```python
from build123d import *

# Parameters (mm, degrees)
F0_R         = 18.561525572
F1_DEPTH     = 25
F2_T         = -2.5
F3_W         = 33.1976041198
F3_H         = 14.1467070207
F4_DEPTH     = 25
F5_T         = -2.5
F7_DEPTH     = 3
F9_DEPTH     = 3
F10_T1_DEPTH = 58.1976041198
F11_T1_DEPTH = 58.1976041198


# Not quite as in the source:
# - a fillet or chamfer that OpenCascade refuses, or shapes differently, is made with other operations: its cross-section is extruded or revolved along the edge and cut away or added
# - a shell that OpenCascade refuses in one call is made with other operations: the cavity is built on its own and cut out


with BuildPart() as f1:
    # F0 (on Top) → F1 (new body)
    with BuildSketch(Plane.XY):
        Circle(F0_R)
    extrude(amount=F1_DEPTH)

    # F2
    f2_openings = [f1.faces().sort_by_distance(p)[0] for p in [
        (0, 0, 25),
        (0, 0, 0),
    ]]
    offset(amount=F2_T, openings=f2_openings)

    # F3 (on Top) → F4 (join)
    with BuildSketch(Plane.XY):
        with Locations((0.0943113118, 0.2829344012)):
            Rectangle(F3_W, F3_H)
    extrude(amount=-F4_DEPTH)

    # F5: a shell. OpenCascade refuses it in one call, so the cavity is built on its own and cut out:
    # the body offset inwards by the wall thickness, plus a prism from it out through each open face.
    f5_core = offset(f1.part, amount=F5_T, mode=Mode.PRIVATE)
    f5_exits = [f5_core.faces().sort_by_distance(p)[0] for p in [
        (0.094311, 0.282934, -22.5),
        (0.094311, 0.282934, -2.5),
    ]]
    add(f5_core, mode=Mode.SUBTRACT)
    extrude(f5_exits, amount=-F5_T, mode=Mode.SUBTRACT)

    # F6 (on Top) → F7 (join)
    with BuildSketch(Plane.XY):
        with BuildLine():
            Line((16.6573040187, -6.7166290246), (-16.5601819754, -6.760219112))
            ThreePointArc((-16.5601819754, -6.760219112), (0.0631717454, -17.8724120589), (16.6573040187, -6.7166290246))
        make_face()
    extrude(amount=F7_DEPTH)

    # F8 (on Top) → F9 (join)
    with BuildSketch(Plane.XY):
        with BuildLine():
            Line((-16.4011158049, 7.3119108565), (16.5623016655, 7.2848270647))
            ThreePointArc((16.5623016655, 7.2848270647), (0.0891507264, 17.7139786602), (-16.4011158049, 7.3119108565))
        make_face()
    extrude(amount=F9_DEPTH)

    # F10: fillet of radius 5 on 1 edges, made by hand

    # F10_s2 → F10_t1 (cut)
    with BuildSketch(Plane.YZ.offset(-29.004490748)):
        with BuildLine():
            ThreePointArc((-1.7904191092, -25), (-5.3259530151, -23.5355339059), (-6.7904191092, -20))
            Line((-6.7904191092, -20), (-6.7904191092, -25))
            Line((-6.7904191092, -25), (-1.7904191092, -25))
        make_face()
    extrude(amount=F10_T1_DEPTH, mode=Mode.SUBTRACT)

    # F11: fillet of radius 5 on 1 edges, made by hand

    # F11_s2 → F11_t1 (cut)
    with BuildSketch(Plane.YZ.offset(-29.004490748)):
        with BuildLine():
            ThreePointArc((7.3562879115, -20), (5.8918218175, -23.5355339059), (2.3562879115, -25))
            Line((2.3562879115, -25), (7.3562879115, -25))
            Line((7.3562879115, -25), (7.3562879115, -20))
        make_face()
    extrude(amount=F11_T1_DEPTH, mode=Mode.SUBTRACT)


solid = f1.part
```
Here's how the part is built. I have some questions about the finished solid (model axes, mm). A direction names the side the tool comes from. Round coordinates to 2 decimals unless told otherwise and drop trailing zeros. Order: outer loops, then holes, each group sorted by start corner. A loop starts at its lowest first (then second) coordinate and runs counter-clockwise, first axis right, second up. Notation, with made-up numbers: (76, 50) -> (103, 50) arc R17 ccw to (103, 58) -> close; hole circle Ø5 at (59.25, 54). An arc over 180 degrees is marked (long way). Use a Markdown table: item, result. Add a question column.
(1) Suppose I cut it at B-B, the plane z = -16. Please give me the cut outline in (x, y).
(2) If we mould it in two halves opening along Y, with no side actions, what happens to faces 1 (the face through (-0.138, -5.854, -22.913)), 2 (the face through (-0.1, 6.5, -22.8)), 3 (the face through (-11, 12, 25)), 4 (the face through (0, -10, 3))? For each: released by +Y, released by -Y, zero draft, split by the parting line, or undercut.
(3) Suppose I cut it at D-D, the plane x = 12. Please give me the cut outline in (y, z).
(4) For pin 1 Ø6 at (x, z) = (-2.5, -5.5) entering from +Y; pin 2 Ø2 at (x, z) = (3, 7.5) entering from -Y; pin 3 Ø2 at (x, z) = (-5, 6) entering from -Y, each with a flat end and sliding along its axis, tell me the tip position at first contact or that it passes through.
(5) Suppose I cut it at C-C, the plane x = 0. Please give me the cut outline in (y, z).
(6) Suppose I cut it at A-A, the plane y = 0. Please give me the cut outline in (x, z), and give its area (3 significant figures).
(7) I need wall thicknesses on line 1 along X through (y, z) = (-2, -16); line 2 along Y through (x, z) = (0, 11.25); line 3 along Y through (x, z) = (10.5, -12). Which ranges of each line are inside material? Lowest first, please.
(8) For faces 5 (the face through (-16.504, 0, -12)), 6 (the face through (-0.2, 5.1, 0)), 7 (the face through (0, 7.356, -10)), which set-ups out of +Z, -Z, +X, -X, +Y, -Y let a thin tool reach every point of the face, with its end or its side?
Verdict:
| question | item | result |
|---|---|---|
| 1 | outline | (-16.5, -6.79) -> (16.69, -6.79) -> (16.69, 7.36) -> (-16.5, 7.36) -> close; hole (-14, -4.29) -> (14.19, -4.29) -> (14.19, 4.86) -> (-14, 4.86) -> close |
| 2 | face 1 | released by -Y |
| 2 | face 2 | released by +Y |
| 2 | face 3 | zero draft |
| 2 | face 4 | undercut |
| 3 | outline | (-14.16, 0) -> (-6.79, 0) -> (-6.79, -20) arc R5 ccw to (-4.29, -24.33) -> (-4.29, 0) -> (-6.72, 0) -> (-6.72, 3) -> (-10.68, 3) -> (-10.68, 25) -> (-14.16, 25) -> close; (4.86, -24.33) arc R5 ccw to (7.36, -20) -> (7.36, 0) -> (14.16, 0) -> (14.16, 25) -> (10.68, 25) -> (10.68, 3) -> (7.29, 3) -> (7.29, 0) -> (4.86, 0) -> close |
| 4 | pin 1 | y = 7.36 |
| 4 | pin 2 | y = -18.45 |
| 4 | pin 3 | y = -18.13 |
| 5 | outline | (-18.56, 0) -> (-6.79, 0) -> (-6.79, -20) arc R5 ccw to (-4.29, -24.33) -> (-4.29, 0) -> (-6.74, 0) -> (-6.74, 3) -> (-16.06, 3) -> (-16.06, 25) -> (-18.56, 25) -> close; (4.86, -24.33) arc R5 ccw to (7.36, -20) -> (7.36, 0) -> (18.56, 0) -> (18.56, 25) -> (16.06, 25) -> (16.06, 3) -> (7.3, 3) -> (7.3, 0) -> (4.86, 0) -> close |
| 6 | outline | (-18.56, 0) -> (-16.5, 0) -> (-16.5, -25) -> (-14, -25) -> (-14, 0) -> (-16.06, 0) -> (-16.06, 25) -> (-18.56, 25) -> close; (14.19, -25) -> (16.69, -25) -> (16.69, 0) -> (18.56, 0) -> (18.56, 25) -> (16.06, 25) -> (16.06, 0) -> (14.19, 0) -> close |
| 6 | area | 250 mm2 |
| 7 | line 1 | -16.5 to -14, 14.19 to 16.69 |
| 7 | line 2 | -18.56 to -16.06, 16.06 to 18.56 |
| 7 | line 3 | -6.79 to -4.29, 4.86 to 7.36 |
| 8 | face 5 | -Z, -X, +Y, -Y |
| 8 | face 6 | +Z |
| 8 | face 7 | -Z, +X, -X, +Y |
